Autodesk Inventor part; units mm, degrees
ref_plane "YZ Plane" through (0, 0, 0) normal (1, 0, 0) x (0, 1, 0)
ref_plane "XZ Plane" through (0, 0, 0) normal (0, 1, 0) x (-1, 0, 0)
ref_plane "XY Plane" through (0, 0, 0) normal (0, 0, 1) x (1, 0, 0)
sketch "Sketch1" plane through (0, 0, 0) normal (0, 0, 1) x (1, 0, 0)
  line L0 (-23.4386, 9.1579) -> (1.5614, 9.1579)
  line L1 (1.5614, 9.1579) -> (1.5614, 5.1579)
  line L2 (1.5614, 5.1579) -> (-23.4386, 5.1579)
  line L3 (-23.4386, 5.1579) -> (-23.4386, 9.1579)
  line L4 (-23.4386, -4.8421) -> (1.5614, -4.8421)
  line L5 (1.5614, -4.8421) -> (1.5614, -8.8421)
  line L6 (1.5614, -8.8421) -> (-23.4386, -8.8421)
  line L7 (-23.4386, -8.8421) -> (-23.4386, -4.8421)
  point P0 (0, 0)
  dimension "d0" = 4
  dimension "d1" = 4
  dimension "d2" = 10
  dimension "d3" = 25
  dimension "d4" = 25
extrude "Extrusion1" add sketch "Sketch1" along normal blind 10
sketch "Sketch2" plane through (0, 0, 0) normal (0, 0, -1) x (-1, 0, 0)
  line L0 (-1.5614, -8.8421) -> (6.4386, -8.8421)
  line L1 (6.4386, -8.8421) -> (6.4386, 9.1579)
  line L2 (6.4386, 9.1579) -> (-1.5614, 9.1579)
  line L3 (-1.5614, 9.1579) -> (-1.5614, -8.8421)
  line L4 (23.4386, 9.1579) -> (-1.5614, 9.1579)
  point P0 (0, 0)
  dimension "d7" = 8
extrude "Extrusion2" add sketch "Sketch2" against normal blind 3
sketch "Sketch3" plane through (-23.4386, -8.8421, 0) normal (0, -1, 0) x (1, 0, 0)
  line L0 (0, 0) -> (0, 10)
  circle A0 centre (5, 5) radius 1.25
  point P0 (23.4386, 0)
  dimension "d10" = 5
  dimension "d11" = 2.5
extrude "Extrusion3" cut sketch "Sketch3" against normal blind 30
chamfer "Chamfer1" distance 2 angle 45 1 edges at (1.5614, 0.1579, 0)
chamfer "Chamfer2" distance 2 angle 45 2 edges at (-23.4386, 7.1579, 10) (-23.4386, -6.8421, 10)
properties part number "Top pully rack"
Can you work these out from the model? Positions are in its coordinate system, mm. A direction names the side the tool comes from. Round coordinates to 2 decimals unless told otherwise and drop trailing zeros. Loops run counter-clockwise (first coordinate to the right, second up) from the corner with the lowest first, then second, coordinate; pieces in that order, holes last.
Item 1: Which directions (+Z, -Z, +X, -X, +Y, -Y) give clear straight access to the entire face, cutting with the end or side of a thin tool? Please do faces 5 (the flat face through (-11, -4.842, 5)), 6 (the flat face through (-22.425, 7.186, 9.014)), 7 (the flat face through (-2, 0, 3)).
Item 2: Suppose I cut it at B-B, the plane z = 5. Write out the boundary of the cut face in (x, y), then the cut area to 3 significant figures.
Item 3: Suppose I cut it at D-D, the plane x = -19. Write out the boundary of the cut face in (y, z), then the cut area to 3 significant figures.
Item 4: Please list where these lines run through material, in increasing order: L1, parallel to Y at x = -21.5, z = 7; L2, parallel to X at y = -7.25, z = 4.5; L3, parallel to Z at x = -4.75, y = -4.
Item 5: Suppose I cut it at A-A, the plane x = -6.75. Write out the boundary of the cut face in (y, z).
Item 6: Will these pins go through, and if not, where does the flat tip stop? pin 1 Ø3 at (x, z) = (-18.44, 5) entering from -Y; pin 2 Ø5 at (y, z) = (-2, 5) entering from -X; pin 3 Ø2.5 at (x, y) = (-1.5, 0.5) entering from +Z; pin 4 Ø1 at (x, y) = (-13, 3) entering from +Z.
Item 7: If we mould it in two halves opening along X, with no side actions, what happens to faces 1 (the cylindrical face through (-18.71, 7.13, 3.78)), 2 (the flat face through (-11, 9.158, 5)), 3 (the cylindrical face through (-18.71, -6.87, 3.78)), 4 (the flat face through (-6.439, 0, 1))? For each: +X half, -X half, draft (parallel to the pull), parting line (faces both ways), or undercut.
Item 8: Suppose I cut it at C-C, the plane y = -6. Write out the boundary of the cut face in (x, z).
Reported:
1. face 5: +Z, -X
1. face 6: +Z, -X, +Y, -Y
1. face 7: +Z, +X, -X
2. outline: (-23.44, -8.84) - (-19.69, -8.84) - (-19.69, -4.84) - (-23.44, -4.84) - close; (-23.44, 5.16) - (-19.69, 5.16) - (-19.69, 9.16) - (-23.44, 9.16) - close; (-17.19, -8.84) - (1.56, -8.84) - (1.56, -4.84) - (-17.19, -4.84) - close; (-17.19, 5.16) - (1.56, 5.16) - (1.56, 9.16) - (-17.19, 9.16) - close
2. area: 180 mm2
3. outline: (-8.84, 0) - (-4.84, 0) - (-4.84, 3.88) - (-8.84, 3.88) - close; (-8.84, 6.12) - (-4.84, 6.12) - (-4.84, 10) - (-8.84, 10) - close; (5.16, 0) - (9.16, 0) - (9.16, 3.88) - (5.16, 3.88) - close; (5.16, 6.12) - (9.16, 6.12) - (9.16, 10) - (5.16, 10) - close
3. area: 62.1 mm2
4. L1: y = -8.84 to -4.84, 5.16 to 9.16
4. L2: x = -23.44 to -19.58, -17.29 to 1.56
4. L3: z = 0 to 3
5. outline: (-8.84, 0) - (-4.84, 0) - (-4.84, 10) - (-8.84, 10) - close; (5.16, 0) - (9.16, 0) - (9.16, 10) - (5.16, 10) - close
6. pin 1: stops at y = -8.84
6. pin 2: stops at x = -6.44
6. pin 3: stops at z = 3
6. pin 4: passes through
7. face 1: undercut
7. face 2: draft
7. face 3: undercut
7. face 4: -X half
8. outline: (-23.44, 0) - (-0.44, 0) - (1.56, 2) - (1.56, 10) - (-21.44, 10) - (-23.44, 8) - close; hole circle Ø2.5 at (-18.44, 5)
